Can you work these out from the model? Positions are in its coordinate system, mm. A direction names the side the tool comes from. Round coordinates to 2 decimals unless told otherwise and drop trailing zeros. Loops run counter-clockwise (first coordinate to the right, second up) from the corner with the lowest first, then second, coordinate; pieces in that order, holes last. Notation, with made-up numbers: M -39,10.25 L -21,10.25 A17 ccw -21,29.25 Z; hole C -37,35.25 d1. An arc over 180 degrees is marked long. Return JSON: item names as keys, results as strings.
```python
from build123d import *

# Parameters (mm, degrees)
SKETCH1_R           = 5.08
BOSS_EXTRUDE1_DEPTH = 133.35
SKETCH2_R           = 3.429
CUT_EXTRUDE1_DEPTH  = 134.35
BOSS_EXTRUDE2_DEPTH = 88.9
HOLE_CUTS_1_REACH   = 12.16
SKETCH4_R           = 1.905
HOLE_CUTS_2_REACH   = 17.219
SKETCH7_R           = 1.905
CUT_EXTRUDE7_REACH  = 135.35
SKETCH8_W           = 6.604
SKETCH8_H           = 4.572
SKETCH9_W           = 11.684
SKETCH9_H           = 88.9
CUT_EXTRUDE8_DEPTH  = 2.54
SKETCH10_W          = 11.684
SKETCH10_H          = 88.9
CUT_EXTRUDE9_DEPTH  = 2.54
SKETCH11_W          = 6.604
SKETCH11_H          = 88.9
CUT_EXTRUDE10_DEPTH = 0.508
SKETCH13_W          = 6.604
SKETCH13_H          = 88.9
CUT_EXTRUDE11_DEPTH = 0.508
SKETCH14_W          = 2.54
SKETCH14_H          = 88.9
BOSS_EXTRUDE3_DEPTH = 1.27
SKETCH15_W          = 2.54
SKETCH15_H          = 88.9
BOSS_EXTRUDE4_DEPTH = 1.27
SKETCH20_W          = 10.0965
SKETCH20_H          = 69.088
CUT_EXTRUDE13_DEPTH = 2.54
SKETCH21_W          = 10.0965
SKETCH21_H          = 69.088
CUT_EXTRUDE14_DEPTH = 2.54


with BuildPart() as part:
    # Sketch1 → Boss-Extrude1 (new body)
    with BuildSketch(Plane(origin=(0, 0, 0), x_dir=(1, 0, 0), z_dir=(0, 1, 0))):
        Circle(SKETCH1_R)
    extrude(amount=BOSS_EXTRUDE1_DEPTH)

    # Sketch2 → Cut-Extrude1 (cut, through all)
    with BuildSketch(Plane.XZ):
        Circle(SKETCH2_R)
    extrude(amount=-CUT_EXTRUDE1_DEPTH, mode=Mode.SUBTRACT)

    # Sketch3 → Boss-Extrude2 (add)
    with BuildSketch(Plane.XZ):
        with BuildLine():
            Line((-1.442590949, 12.658640818), (-5.842, 10.118640818))
            Line((-5.842, 10.118640818), (-2.54, 4.399409051))
            ThreePointArc((-2.54, 4.399409051), (2.96960111, -1.7145), (-5.08, 0))
            Line((-5.08, 0), (-11.684, 0))
            Line((-11.684, 0), (-11.684, -5.08))
            Line((-11.684, -5.08), (-11.684, -10.16))
            Line((-11.684, -10.16), (0, -10.16))
            Line((0, -10.16), (0, -5.08))
            ThreePointArc((0, -5.08), (4.399409051, -2.54), (4.399409051, 2.54))
            Line((4.399409051, 2.54), (8.798818102, 5.08))
            Line((8.798818102, 5.08), (2.956818102, 15.198640818))
            Line((2.956818102, 15.198640818), (-1.442590949, 12.658640818))
        make_face()
    extrude(amount=-BOSS_EXTRUDE2_DEPTH)

    # Sketch4 → Hole Cuts 1 (cut, up to next)
    with BuildSketch(Plane.XY, mode=Mode.PRIVATE) as hole_cuts_1_sk1:
        with Locations((-8.89, 80.01)):
            Circle(SKETCH4_R)
    hole_cuts_1_tool1 = extrude(hole_cuts_1_sk1.sketch, amount=-HOLE_CUTS_1_REACH, mode=Mode.PRIVATE) & part.part
    add(hole_cuts_1_tool1.solids().sort_by_distance((-8.89, 80.01, 0))[0], mode=Mode.SUBTRACT)
    # Sketch4 → Hole Cuts 1 (cut, up to next)
    with BuildSketch(Plane.XY, mode=Mode.PRIVATE) as hole_cuts_1_sk2:
        with Locations((-8.89, 3.81)):
            Circle(SKETCH4_R)
    hole_cuts_1_tool2 = extrude(hole_cuts_1_sk2.sketch, amount=-HOLE_CUTS_1_REACH, mode=Mode.PRIVATE) & part.part
    add(hole_cuts_1_tool2.solids().sort_by_distance((-8.89, 3.81, 0))[0], mode=Mode.SUBTRACT)

    # Sketch7 → Hole Cuts 2 (cut, up to next)
    with BuildSketch(Plane(origin=(0, 0, 0), x_dir=(0.5, 0, -0.866025404), z_dir=(0.866025404, 0, 0.5)), mode=Mode.PRIVATE) as hole_cuts_2_sk1:
        with Locations((-8.89, 85.09)):
            Circle(SKETCH7_R)
    hole_cuts_2_tool1 = extrude(hole_cuts_2_sk1.sketch, amount=HOLE_CUTS_2_REACH, mode=Mode.PRIVATE) & part.part
    add(hole_cuts_2_tool1.solids().sort_by_distance((-4.445, 85.09, 7.698966))[0], mode=Mode.SUBTRACT)
    # Sketch7 → Hole Cuts 2 (cut, up to next)
    with BuildSketch(Plane(origin=(0, 0, 0), x_dir=(0.5, 0, -0.866025404), z_dir=(0.866025404, 0, 0.5)), mode=Mode.PRIVATE) as hole_cuts_2_sk2:
        with Locations((-8.89, 8.255)):
            Circle(SKETCH7_R)
    hole_cuts_2_tool2 = extrude(hole_cuts_2_sk2.sketch, amount=HOLE_CUTS_2_REACH, mode=Mode.PRIVATE) & part.part
    add(hole_cuts_2_tool2.solids().sort_by_distance((-4.445, 8.255, 7.698966))[0], mode=Mode.SUBTRACT)

    # Sketch8 → Cut-Extrude7 (cut, up to next)
    with BuildSketch(Plane.XZ, mode=Mode.PRIVATE) as cut_extrude7_sk1:
        Polygon((-5.842, 10.118640818), (-1.882531854, 12.404640818), (1.419468146, 6.685409051), (-2.54, 4.399409051), align=None)
    cut_extrude7_tool1 = extrude(cut_extrude7_sk1.sketch, amount=-CUT_EXTRUDE7_REACH, mode=Mode.PRIVATE) & part.part
    add(cut_extrude7_tool1.solids().sort_by_distance((-2.211266, 0, 8.402025))[0], mode=Mode.SUBTRACT)
    # Sketch8 → Cut-Extrude7 (cut, up to next)
    with BuildSketch(Plane.XZ, mode=Mode.PRIVATE) as cut_extrude7_sk2:
        with Locations((-8.382, -2.286)):
            Rectangle(SKETCH8_W, SKETCH8_H)
    cut_extrude7_tool2 = extrude(cut_extrude7_sk2.sketch, amount=-CUT_EXTRUDE7_REACH, mode=Mode.PRIVATE) & part.part
    add(cut_extrude7_tool2.solids().sort_by_distance((-8.382, 0, -2.286))[0], mode=Mode.SUBTRACT)

    # Sketch9 → Cut-Extrude8 (cut)
    with BuildSketch(Plane(origin=(0, 0, -10.16), x_dir=(-1, 0, 0), z_dir=(0, 0, -1))):
        with Locations((5.842, 44.45)):
            Rectangle(SKETCH9_W, SKETCH9_H)
    extrude(amount=-CUT_EXTRUDE8_DEPTH, mode=Mode.SUBTRACT)

    # Sketch10 → Cut-Extrude9 (cut)
    with BuildSketch(Plane(origin=(8.798818102, 0, 5.08), x_dir=(0.5, 0, -0.866025404), z_dir=(0.866025404, 0, 0.5))):
        with Locations((-5.842, 44.45)):
            Rectangle(SKETCH10_W, SKETCH10_H)
    extrude(amount=-CUT_EXTRUDE9_DEPTH, mode=Mode.SUBTRACT)

    # Sketch11 → Cut-Extrude10 (cut)
    with BuildSketch(Plane.XY.offset(-4.572)):
        with Locations((-8.382, 44.45)):
            Rectangle(SKETCH11_W, SKETCH11_H)
    extrude(amount=-CUT_EXTRUDE10_DEPTH, mode=Mode.SUBTRACT)

    # Sketch13 → Cut-Extrude11 (cut)
    with BuildSketch(Plane(origin=(3.959468146, 0, 2.286), x_dir=(-0.5, 0, 0.866025404), z_dir=(-0.866025404, 0, -0.5))):
        with Locations((8.382, 44.45)):
            Rectangle(SKETCH13_W, SKETCH13_H)
    extrude(amount=-CUT_EXTRUDE11_DEPTH, mode=Mode.SUBTRACT)

    # Sketch14 → Boss-Extrude3 (add)
    with BuildSketch(Plane(origin=(-5.842, 0, 10.118640818), x_dir=(0.866025404, 0, 0.5), z_dir=(-0.5, 0, 0.866025404))):
        with Locations((6.35, 44.45)):
            Rectangle(SKETCH14_W, SKETCH14_H)
    extrude(amount=BOSS_EXTRUDE3_DEPTH)

    # Sketch15 → Boss-Extrude4 (add)
    with BuildSketch(Plane.ZY.offset(11.684)):
        with Locations((-6.35, 44.45)):
            Rectangle(SKETCH15_W, SKETCH15_H)
    extrude(amount=BOSS_EXTRUDE4_DEPTH)

    # Sketch20 → Cut-Extrude13 (cut)
    with BuildSketch(Plane.XY.offset(-5.08)):
        with Locations((-7.90575, 41.91)):
            Rectangle(SKETCH20_W, SKETCH20_H)
    extrude(amount=-CUT_EXTRUDE13_DEPTH, mode=Mode.SUBTRACT)

    # Sketch21 → Cut-Extrude14 (cut)
    with BuildSketch(Plane(origin=(6.599113577, 0, 3.81), x_dir=(0.5, 0, -0.866025404), z_dir=(0.866025404, 0, 0.5))):
        with Locations((-7.90575, 46.6725)):
            Rectangle(SKETCH21_W, SKETCH21_H)
    extrude(amount=-CUT_EXTRUDE14_DEPTH, mode=Mode.SUBTRACT)


solid = part.part
```
Q1. If I drill on line 1 along Y through (x, z) = (2, 11.25); line 2 along Y through (x, z) = (3, 6.75); line 3 along X through (y, z) = (80.01, -6.65) (3 decimals), over which ranges is the centre line in solid material (lowest first)?
Results:
{"line 1": "y = 0 to 6.36, 10.15 to 12.13, 81.22 to 83.19, 86.99 to 88.9", "line 2": "y = 0 to 12.13, 81.22 to 88.9", "line 3": "x = -12.954 to -10.795, -6.985 to 0"}
Q2. I'm going to push flat-ended pins straight in: pin 1 Ø5 at (y, z) = (52.5, 5) entering from +X; pin 2 Ø1.5 at (x, y) = (-1.5, 109) entering from -Z; pin 3 Ø9 at (x, z) = (0, 0) entering from +Y; pin 4 Ø3 at (y, z) = (54.5, -7) entering from -X. Where does each tip first touch, or does it pass through?
Results:
{"pin 1": "stops at x = 6.6", "pin 2": "stops at z = -5.02", "pin 3": "stops at y = 133.35", "pin 4": "stops at x = -2.86"}
Q3. Suppose I cut it at C-C, the plane y = 70.5. Please give me the cut outline in (x, z).
Results:
{"outline": "M -5.08,-5.08 L -2.86,-5.08 L -2.86,-7.62 L 0,-7.62 L 0,-5.08 A5.08 ccw 4.4,2.54 L 6.6,3.81 L 5.17,6.28 L 2.97,5.01 L 1.86,6.94 L -2.54,4.4 A5.08 ccw -5.08,0 Z; hole C 0,0 d6.86"}
Q4. Suppose I cut it at D-D, the plane y = 112.5. Please give me the cut outline in (x, z).
Results:
{"outline": "C 0,0 d10.16; hole C 0,0 d6.86"}
Q5. Suppose I cut it at B-B, the plane x = -8.89. Please give me the cut outline in (y, z) (3 decimals), plus the area to 3 significant figures.
Results:
{"outline": "M 0,-7.62 L 1.905,-7.62 L 1.905,-5.08 L 0,-5.08 Z; M 5.715,-7.62 L 7.366,-7.62 L 7.366,-5.08 L 5.715,-5.08 Z; M 76.454,-7.62 L 78.105,-7.62 L 78.105,-5.08 L 76.454,-5.08 Z; M 81.915,-7.62 L 88.9,-7.62 L 88.9,-5.08 L 81.915,-5.08 Z", "area": "31.0 mm2"}
Q6. On a 3-axis mill with a long thin cutter (end or side, diameter ignored), from which of +Z, -Z, +X, -X, +Y, -Y can I reach the whole of each face in a straight line? I mean faces 1 (the flat face through (-9, 83, -5.08)), 2 (the flat face through (-0.96, 83.3, 11.82)), 3 (the flat face through (0, 44, -6)). Say none if no direction works.
Results:
{"face 1": "+Z, -X, +Y, -Y", "face 2": "-X, +Y, -Y", "face 3": "-Z, +X, +Y, -Y"}
Q7. Suppose I cut it at A-A, the plane y = 3.81. Please give me the cut outline in (x, z) (1 decimal).
Results:
{"outline": "M -13,-7.6 L -10.8,-7.6 L -10.8,-5.1 L -13,-5.1 Z; M -7,-7.6 L 0,-7.6 L 0,-5.1 A5.1 ccw 4.4,2.5 L 6.6,3.8 L 0.1,15 L -2.1,13.8 L 1.9,6.9 L -2.5,4.4 A5.1 ccw -5.1,0 L -5.1,-5.1 L -7,-5.1 Z; hole C 0,0 d6.9"}
Q8. Thinking about a two-plate mould opening in Y: for faces 4 (the flat face through (-3, 0, 2)), 5 (the flat face through (-12.954, 4, -6)), 6 (the flat face through (-2.858, 41, -6)), which applies, pulls with the +Y half, pulls with the -Y half, needs draft (parallel to the pull), parting line crosses it, or undercut?
Results:
{"face 4": "pulls with the -Y half", "face 5": "needs draft", "face 6": "undercut"}
